```python
from build123d import *

# Parameters (mm, degrees)
BASE_FLANGE1_OUTLINE_W = 10
BASE_FLANGE1_OUTLINE_H = 140
BASE_FLANGE1_DEPTH     = 300
SKETCH6_R              = 2.5
CUT_EXTRUDE1_DEPTH     = 10
SKETCH11_R             = 1.5
CUT_EXTRUDE2_DEPTH     = 10
CUT_EXTRUDE3_DEPTH     = 10


# Read off the part's stored shape, not the designer's step: Base-Flange1
with BuildPart() as part:
    # Base-Flange1 outline → Base-Flange1 (new body)
    with BuildSketch(Plane(origin=(0, 0, 0), x_dir=(1, 0, 0), z_dir=(0, 1, 0))):
        with Locations((-5, 0)):
            Rectangle(BASE_FLANGE1_OUTLINE_W, BASE_FLANGE1_OUTLINE_H)
    extrude(amount=BASE_FLANGE1_DEPTH)

    # Sketch6 → Cut-Extrude1 (cut)
    with BuildSketch(Plane.ZY.offset(10)):
        with Locations((57.5, 10)):
            Circle(SKETCH6_R)
        with Locations((-57.5, 10)):
            Circle(SKETCH6_R)
        with Locations((-57.5, 50)):
            Circle(SKETCH6_R)
        with Locations((57.5, 50)):
            Circle(SKETCH6_R)
        with Locations(Location((57.5, 250, 0), (0, 0, 180))):
            Circle(SKETCH6_R)
        with Locations(Location((-57.5, 250, 0), (0, 0, 180))):
            Circle(SKETCH6_R)
        with Locations(Location((-57.5, 290, 0), (0, 0, 180))):
            Circle(SKETCH6_R)
        with Locations(Location((57.5, 290, 0), (0, 0, 180))):
            Circle(SKETCH6_R)
    extrude(amount=-CUT_EXTRUDE1_DEPTH, mode=Mode.SUBTRACT)

    # Sketch11 → Cut-Extrude2 (cut)
    with BuildSketch(Plane(origin=(0, 0, 0), x_dir=(0, 0, -1), z_dir=(1, 0, 0))):
        with Locations((57.5, 220)):
            Circle(SKETCH11_R)
        with Locations((-57.5, 220)):
            Circle(SKETCH11_R)
        with Locations((-57.5, 70)):
            Circle(SKETCH11_R)
        with Locations((57.5, 70)):
            Circle(SKETCH11_R)
    extrude(amount=-CUT_EXTRUDE2_DEPTH, mode=Mode.SUBTRACT)

    # Sketch12 → Cut-Extrude3 (cut)
    with BuildSketch(Plane.ZY.offset(10)):
        with BuildLine():
            Line((60, 206.940043573), (60, 176.940043573))
            ThreePointArc((60, 176.940043573), (57.5, 174.440043573), (55, 176.940043573))
            Line((55, 176.940043573), (55, 206.940043573))
            ThreePointArc((55, 206.940043573), (57.5, 209.440043573), (60, 206.940043573))
        make_face()
        with BuildLine():
            Line((-55, 206.940043573), (-55, 176.940043573))
            ThreePointArc((-55, 176.940043573), (-57.5, 174.440043573), (-60, 176.940043573))
            Line((-60, 176.940043573), (-60, 206.940043573))
            ThreePointArc((-60, 206.940043573), (-57.5, 209.440043573), (-55, 206.940043573))
        make_face()
        with BuildLine():
            Line((-55, 111.940043573), (-55, 81.940043573))
            ThreePointArc((-55, 81.940043573), (-57.5, 79.440043573), (-60, 81.940043573))
            Line((-60, 81.940043573), (-60, 111.940043573))
            ThreePointArc((-60, 111.940043573), (-57.5, 114.440043573), (-55, 111.940043573))
        make_face()
        with BuildLine():
            Line((60, 111.940043573), (60, 81.940043573))
            ThreePointArc((60, 81.940043573), (57.5, 79.440043573), (55, 81.940043573))
            Line((55, 81.940043573), (55, 111.940043573))
            ThreePointArc((55, 111.940043573), (57.5, 114.440043573), (60, 111.940043573))
        make_face()
    extrude(amount=-CUT_EXTRUDE3_DEPTH, mode=Mode.SUBTRACT)


solid = part.part
```
Design review of the part built by this model. Coordinates are the model's own, in mm. A direction names the side the tool comes from. Round coordinates to 2 decimals unless told otherwise and drop trailing zeros. Write each loop counter-clockwise with the first axis right and the second up, starting at its lowest first coordinate (ties: lowest second). Pieces come first, ordered by that corner, then holes.
Item 1: For probe 1 along Z at (x, y) = (-7.5, 250); probe 2 along Z at (x, y) = (-4, 220), list the stretches that pass through material, from the lowest coordinate up.
Item 2: For faces 4 (the flat face through (-5, 148, -70)), 5 (the cylindrical face through (-5.07, 174.44, 57.55)), list the 3-axis set-ups (+Z, -Z, +X, -X, +Y, -Y) from which the entire face can be reached by the end or side of a thin tool; tool diameter is ignored.
Item 3: We need section B-B on y = 199. Write out the cut boundary in (x, z).
Item 4: Clearance check with a flat-ended pin moving along its axis: pin 1 Ø4 at (y, z) = (250, -57.5) entering from +X. State where the tip first meets the part, or that it passes through.
Item 5: We need section A-A on x = -5.25. State how many separate pieces and enclosed holes the cut face has, and give its area (3 significant figures).
Item 6: The part is to be moulded in two halves that separate along Y. For faces 1 (the flat face through (-5, 192, 60)), 2 (the flat face through (-5, 148, 70)), 3 (the flat face through (-5, 0, -1)), say which applies: +Y half, -Y half, draft (parallel to the pull), parting line (faces both ways), or undercut.
Returned:
1. probe 1: z = -70 to -60, -55 to 55, 60 to 70
1. probe 2: z = -70 to -59, -56 to 56, 59 to 70
2. face 4: -Z, +X, -X, +Y, -Y
2. face 5: +X, -X
3. outline: (-10, -70) - (0, -70) - (0, -60) - (-10, -60) - close; (-10, -55) - (0, -55) - (0, 55) - (-10, 55) - close; (-10, 60) - (0, 60) - (0, 70) - (-10, 70) - close
4. pin 1: passes through
5. separate pieces: 1
5. enclosed holes: 16
5. area: 41,100 mm2
6. face 1: undercut
6. face 2: draft
6. face 3: -Y half
